Autodesk Inventor part; units mm, degrees
ref_plane "YZ Plane" through (0, 0, 0) normal (1, 0, 0) x (0, 1, 0)
ref_plane "XZ Plane" through (0, 0, 0) normal (0, 1, 0) x (-1, 0, 0)
ref_plane "XY Plane" through (0, 0, 0) normal (0, 0, 1) x (1, 0, 0)
sketch "Sketch1" plane through (0, 0, 0) normal (0, 0, 1) x (1, 0, 0)
  line L0 (0, 0) -> (-5, 0)
  line L1 (-5, 0) -> (-5, 2.5)
  line L2 (-5, 2.5) -> (-10, 2.5)
  line L3 (-10, 2.5) -> (-10, 7.5)
  line L4 (-10, 7.5) -> (-5, 7.5)
  line L5 (-5, 7.5) -> (-5, 12.5)
  line L6 (-5, 12.5) -> (0, 12.5)
  line L7 (-5, 0) -> (-5, -2.5)
  line L8 (-5, -2.5) -> (-10, -2.5)
  line L9 (-10, -2.5) -> (-10, -7.5)
  line L10 (-10, -7.5) -> (-5, -7.5)
  line L11 (-5, -7.5) -> (-5, -12.5)
  line L12 (-5, -12.5) -> (0, -12.5)
  line L13 (0, 12.5) -> (0, 17.5)
  line L14 (0, 17.5) -> (5, 17.5)
  line L15 (5, 17.5) -> (5, 12.5)
  line L16 (5, 12.5) -> (10, 12.5)
  line L17 (10, 12.5) -> (10, 17.5)
  line L18 (10, 17.5) -> (15, 17.5)
  line L19 (15, 17.5) -> (15, 12.5)
  line L20 (15, 12.5) -> (20, 12.5)
  line L21 (20, 12.5) -> (20, 7.5)
  line L22 (20, 7.5) -> (25, 7.5)
  line L23 (25, 7.5) -> (25, 2.5)
  line L24 (25, 2.5) -> (20, 2.5)
  line L25 (20, 2.5) -> (20, -2.5)
  line L26 (20, -2.5) -> (25, -2.5)
  line L27 (25, -2.5) -> (25, -7.5)
  line L28 (25, -7.5) -> (20, -7.5)
  line L29 (20, -7.5) -> (20, -12.5)
  line L30 (20, -12.5) -> (15, -12.5)
  line L31 (15, -12.5) -> (15, -17.5)
  line L32 (15, -17.5) -> (10, -17.5)
  line L33 (10, -17.5) -> (10, -12.5)
  line L34 (10, -12.5) -> (5, -12.5)
  line L35 (5, -12.5) -> (5, -17.5)
  line L36 (5, -17.5) -> (0, -17.5)
  line L37 (0, -17.5) -> (0, -12.5)
  line L38 (0, 17.5) -> (-10, 17.5)
  line L39 (-10, 17.5) -> (-10, 7.5)
  line L40 (15, 17.5) -> (25, 17.5)
  line L41 (25, 17.5) -> (25, 7.5)
  line L42 (25, -7.5) -> (25, -17.5)
  line L43 (25, -17.5) -> (15, -17.5)
  line L44 (0, -17.5) -> (-10, -17.5)
  line L45 (-10, -7.5) -> (-10, -17.5)
  dimension "d0" = 5
  dimension "d1" = 2.5
  dimension "d2" = 5
  dimension "d3" = 5
  dimension "d4" = 5
  dimension "d5" = 5
  dimension "d6" = 5
  dimension "d7" = 2.5
  dimension "d8" = 5
  dimension "d9" = 5
  dimension "d10" = 5
  dimension "d11" = 5
  dimension "d12" = 5
  dimension "d13" = 5
  dimension "d14" = 5
  dimension "d15" = 5
  dimension "d16" = 5
  dimension "d17" = 5
  dimension "d18" = 5
  dimension "d19" = 5
  dimension "d20" = 5
  dimension "d21" = 5
  dimension "d22" = 5
  dimension "d23" = 5
  dimension "d24" = 5
  dimension "d25" = 5
  dimension "d26" = 5
  dimension "d27" = 5
  dimension "d28" = 5
  dimension "d29" = 5
  dimension "d30" = 5
  dimension "d31" = 5
  dimension "d32" = 5
extrude "Extrusion1" add sketch "Sketch1" along normal blind 5
sketch "Sketch4" plane through (0, 0, 5) normal (0, 0, 1) x (1, 0, 0)
  line L0 (-10, 17.5) -> (-10, 13.5)
  line L1 (-10, 17.5) -> (-10, 2.5)
  line L2 (-10, 13.5) -> (-6, 13.5)
  circle A0 centre (-6, 13.5) radius 1.75
  point P0 (0, 0)
  dimension "d54" = 4
  dimension "d55" = 4
  dimension "d56" = 3.5
extrude "Extrusion4" cut sketch "Sketch4" against normal blind 10
sketch "Sketch5" plane through (0, 0, 5) normal (0, 0, 1) x (1, 0, 0)
  circle A0 centre (-6, 13.5) radius 1.75
  line L0 (-6, 13.5) -> (-3, 13.5)
  line L1 (-3, 13.5) -> (-4.5, 16.0981)
  line L2 (-4.5, 16.0981) -> (-6, 13.5)
  point P0 (0, 0)
  dimension "d59" = 3
  dimension "d60" = 3
  dimension "d61" = 60
extrude "Extrusion5" cut sketch "Sketch5" against normal blind 2.5 contours L0 L2 A0 | A0 L2 L1 L0 picked at (-4.9952, 14.0801)
pattern_circular "Circular Pattern2" count 6 over 360 about axis through (-6, 13.5, 5) along (0, 0, -1) of "Extrusion5"
sketch "Sketch6" plane through (0, 0, 5) normal (0, 0, 1) x (1, 0, 0)
  line L0 (-5, -2.5) -> (-5, 2.5)
  line L1 (-5, 0) -> (20, 0)
  line L2 (20, 2.5) -> (20, -2.5)
  line L3 (5, 12.5) -> (10, 12.5)
  line L4 (7.5, 12.5) -> (7.5, 0)
  circle A0 centre (7.5, 0) radius 7
  point P0 (0, 0)
  dimension "d70" = 14
extrude "Extrusion6" cut sketch "Sketch6" against normal through all
pattern_circular "Circular Pattern4" count 4 over 360 about axis through (7.5, 0, 5) along (0, 0, -1) of "Extrusion5", "Circular Pattern2", "Extrusion4"
properties part number "crossCenter"
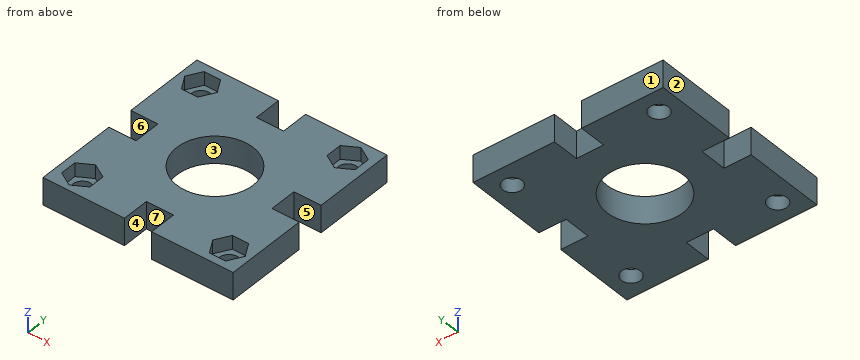
Geometry: final body of the model. Coordinates: model frame, mm. Face numbers are marked on the shaded views. A direction names the side the tool comes from. Coordinates: 2 decimals unless noted, no trailing zeros. Order: outer loops, then holes, each group sorted by start corner. A loop starts at its lowest first (then second) coordinate and runs counter-clockwise, first axis right, second up.
(1) Section query D-D (z = 3.95). State how many separate pieces and enclosed holes the cut face has, plus the area to 3 significant figures.
(2) Section query B-B (y = -1). Return the cut outline in (x, z), plus the area to 3 significant figures.
(3) Access query for the marked faces 5, 6 and 7. Directions: +Z, -Z, +X, -X, +Y, -Y. A direction counts if a zero-diameter tool reaches every point of the face in a straight line with its end or side. Return the directions, or none.
(4) First-contact query: pin 1 (2.5 mm diameter, centred on x = 20.5, y = -14, fed in from +Z); pin 2 (2 mm diameter, centred on x = 7.5, z = 2.5, fed in from -Y); pin 3 (3 mm diameter, centred on x = -6, y = -13.5, fed in from -Z). Flat tips, straight axial feed; report the tip coordinate or a pass-through.
(5) Draft query along X for the marked faces 1, 2, 3 and 4. Return one class per face: pulls with the +X half, pulls with the -X half, needs draft (parallel to the pull), parting line crosses it, or undercut.
(6) Material intervals for probe 1 along Y at (x, z) = (-6, 0.6); probe 2 along X at (y, z) = (-13.5, 0.9); probe 3 along X at (y, z) = (0, 3.7), sorted ascending.
(7) Section query A-A (x = 7.5). Return the cut outline in (y, z), plus the area to 3 significant figures.
(8) Section query C-C (z = 1.55). Return the cut outline in (x, y).
Solution:
1. separate pieces: 1
1. enclosed holes: 5
1. area: 878 mm2
2. outline: (-5, 0) - (0.57, 0) - (0.57, 5) - (-5, 5) - close; (14.43, 0) - (20, 0) - (20, 5) - (14.43, 5) - close
2. area: 55.7 mm2
3. face 5: +Z, -Z, +X
3. face 6: +Z, -Z, -X
3. face 7: +Z, -Z, -Y
4. pin 1: stops at z = 2.5
4. pin 2: stops at y = -12.5
4. pin 3: passes through
5. face 1: needs draft
5. face 2: pulls with the -X half
5. face 3: undercut
5. face 4: undercut
6. probe 1: y = -17.5 to -15.25, -11.75 to -2.5, 2.5 to 11.75, 15.25 to 17.5
6. probe 2: x = -10 to -7.75, -4.25 to 5, 10 to 19.25, 22.75 to 25
6. probe 3: x = -5 to 0.5, 14.5 to 20
7. outline: (-12.5, 0) - (-7, 0) - (-7, 5) - (-12.5, 5) - close; (7, 0) - (12.5, 0) - (12.5, 5) - (7, 5) - close
7. area: 55.0 mm2
8. outline: (-10, -17.5) - (5, -17.5) - (5, -12.5) - (10, -12.5) - (10, -17.5) - (25, -17.5) - (25, -2.5) - (20, -2.5) - (20, 2.5) - (25, 2.5) - (25, 17.5) - (10, 17.5) - (10, 12.5) - (5, 12.5) - (5, 17.5) - (-10, 17.5) - (-10, 2.5) - (-5, 2.5) - (-5, -2.5) - (-10, -2.5) - close; hole circle Ø3.5 at (-6, -13.5); hole circle Ø3.5 at (-6, 13.5); hole circle Ø14 at (7.5, 0); hole circle Ø3.5 at (21, -13.5); hole circle Ø3.5 at (21, 13.5)
